Check sheet for the modelled part. Datum: model origin and axes. Units: mm. Face numbers are marked on the shaded views. A direction names the side the tool comes from. Round coordinates to 2 decimals unless told otherwise and drop trailing zeros. Order: outer loops, then holes, each group sorted by start corner. A loop starts at its lowest first (then second) coordinate and runs counter-clockwise, first axis right, second up.
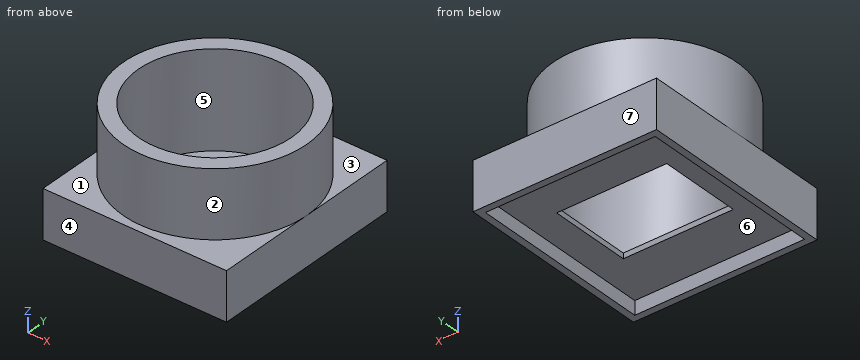
```python
from build123d import *

# Parameters (mm, degrees)
F0_W     = 12
F0_H     = 13
F0_W_2   = 11.1
F0_H_2   = 12.1
F0_W_3   = 7.2
F0_H_3   = 5.4
F1_DEPTH = 3.15
F2_DEPTH = 0.9
F3_R     = 5
F4_DEPTH = 4.35
F5_DEPTH = 1.9


with BuildPart() as f1:
    # F0 (on Top) → F1 (new body)
    with BuildSketch(Plane.XY):
        Rectangle(F0_W, F0_H)
        Rectangle(F0_W_2, F0_H_2, mode=Mode.SUBTRACT)
        Rectangle(F0_W_2, F0_H_2)
        Rectangle(F0_W_3, F0_H_3, mode=Mode.SUBTRACT)
    extrude(amount=F1_DEPTH)

    # F0 (on Top) → F2 (cut)
    with BuildSketch(Plane.XY):
        Rectangle(F0_W_2, F0_H_2)
        Rectangle(F0_W_3, F0_H_3, mode=Mode.SUBTRACT)
    extrude(amount=F2_DEPTH, mode=Mode.SUBTRACT)

    # F3 (on face) → F4 (join)
    with BuildSketch(Plane.XY.offset(3.15)):
        with BuildLine():
            ThreePointArc((-6, 0), (0, -6), (6, 0))
            ThreePointArc((6, 0), (0, 6), (-6, 0))
        make_face()
        Circle(F3_R, mode=Mode.SUBTRACT)
    extrude(amount=F4_DEPTH)

    # F5 (cut): a face of the model
    f5_faces = [f1.faces().sort_by_distance(p)[0] for p in [
        (-4.8585786438, 0, 3.15),
    ]]
    extrude(f5_faces, amount=-F5_DEPTH, mode=Mode.SUBTRACT)


solid = f1.part
```
Item 1: Release check for a two-part mould opening along Y. For the marked faces 4, 5, 6 and 7 record: released by +Y, released by -Y, zero draft, split by the parting line, or undercut.
Answer:
face 4: released by -Y
face 5: undercut
face 6: undercut
face 7: released by +Y
Item 2: Sectioned sample at D-D (x = -4). Record the cut outline in (y, z), and give its area (3 significant figures).
Answer:
outline: (-6.5, 0) - (-6.05, 0) - (-6.05, 0.9) - (6.05, 0.9) - (6.05, 0) - (6.5, 0) - (6.5, 3.15) - (4.47, 3.15) - (4.47, 7.5) - (3, 7.5) - (3, 1.25) - (-3, 1.25) - (-3, 7.5) - (-4.47, 7.5) - (-4.47, 3.15) - (-6.5, 3.15) - close
area: 31.5 mm2
Item 3: Sectioned sample at C-C (z = 2.25). Record the cut outline in (x, y).
Answer:
outline: (-6, -6.5) - (6, -6.5) - (6, 6.5) - (-6, 6.5) - close; hole circle Ø10 at (0, 0)
Item 4: Sectioned sample at A-A (x = 0). Record the cut outline in (y, z), and give its area (3 significant figures).
Answer:
outline: (-6.5, 0) - (-6.05, 0) - (-6.05, 0.9) - (-2.7, 0.9) - (-2.7, 1.25) - (-5, 1.25) - (-5, 7.5) - (-6, 7.5) - (-6, 3.15) - (-6.5, 3.15) - close; (2.7, 0.9) - (6.05, 0.9) - (6.05, 0) - (6.5, 0) - (6.5, 3.15) - (6, 3.15) - (6, 7.5) - (5, 7.5) - (5, 1.25) - (2.7, 1.25) - close
area: 17.9 mm2
Item 5: Go/stop test with flat-tipped pins: P1, Ø1, axis at x = -4, z = 5.5, coming from the +Y side; P2, Ø2, axis at x = -2, y = 3, coming from the +Z side; P3, Ø3, axis at x = -3, y = 0.5, coming from the -Z side; P4, Ø5, axis at x = -1, y = -3, coming from the +Z side. Record where each tip stops, or that it passes through.
Answer:
P1: stops at y = 4.87
P2: stops at z = 1.25
P3: stops at z = 0.9
P4: stops at z = 7.5
Item 6: Access from +Z, -Z, +X, -X, +Y, -Y to the whole of each face (thin tool, end or side, straight path). Record for the marked faces 1, 2 and 3.
Answer:
face 1: +Z, -Y
face 2: +Z
face 3: +Z, +Y
Item 7: Scan lines: line 1 along Y through (x, z) = (0, 2.75); line 2 along Y through (x, z) = (0, 6.25); line 3 along Z through (x, y) = (5.5, 0.25). Record each from-to range of solid material in increasing order.
Answer:
line 1: y = -6.5 to -5, 5 to 6.5
line 2: y = -6 to -5, 5 to 6
line 3: z = 0.9 to 7.5
Item 8: Sectioned sample at B-B (y = -2.5). Record the cut outline in (x, z).
Answer:
outline: (-6, 0) - (-5.55, 0) - (-5.55, 0.9) - (-3.6, 0.9) - (-3.6, 1.25) - (-4.33, 1.25) - (-4.33, 7.5) - (-5.45, 7.5) - (-5.45, 3.15) - (-6, 3.15) - close; (3.6, 0.9) - (5.55, 0.9) - (5.55, 0) - (6, 0) - (6, 3.15) - (5.45, 3.15) - (5.45, 7.5) - (4.33, 7.5) - (4.33, 1.25) - (3.6, 1.25) - close
